Check sheet for the drawn part. Datum: minimum x, y, z corner. Units: mm. Coordinates: 2 decimals unless noted, no trailing zeros. Write each loop counter-clockwise with the first axis right and the second up, starting at its lowest first coordinate (ties: lowest second). Pieces come first, ordered by that corner, then holes. Notation, with made-up numbers: (-33, 88.25) -> (-19, 88.25) arc R29 cw to (-19, 116.25) -> close; hole circle Ø1 at (28.25, -24.75). An arc over 180 degrees is marked (long way). Answer in a Markdown table with one row per item. Add a question column.
Q1. Release check for a two-part mould opening along X. For the marked faces 1 and 2 record: pulls with the +X half, pulls with the -X half, needs draft (parallel to the pull), parting line crosses it, or undercut.
Q2. Section check C-C, the plane x = 30. Record the boundary of the cut face in (y, z) (1 decimal).
Q3. Section check D-D, the plane z = 1.5. Record the boundary of the cut face in (x, y) (1 decimal).
Q4. Thickness scan on line 1 (X direction, y = 12, z = 2.2) (1 decimal); line 2 (Y direction, x = 43, z = 0.35); line 3 (Y direction, x = 30, z = 2.8) (1 decimal). Record the ranges inside material, lowest first.
Q5. Gauge pin test, flat end, axial feed: P1, Ø8.5, axis at x = 29, y = 10, coming from the +Z side. Record the tip position at first contact, or that the pin passes through.
Q6. Section check A-A, the plane x = 43. Record the boundary of the cut face in (y, z).
Q7. Section check B-B, the plane y = 12. Record the boundary of the cut face in (x, z) (1 decimal).
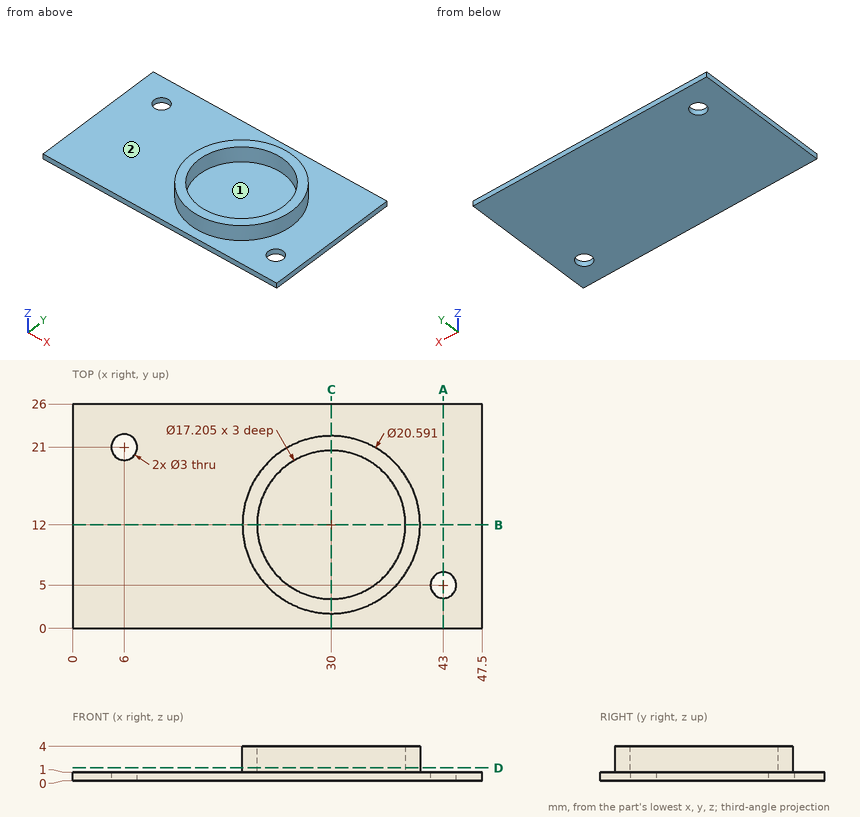
Calculated:
| question | item | result |
|---|---|---|
| 1 | face 1 | undercut |
| 1 | face 2 | needs draft |
| 2 | outline | (0, 0) -> (26, 0) -> (26, 1) -> (22.3, 1) -> (22.3, 4) -> (20.6, 4) -> (20.6, 1) -> (3.4, 1) -> (3.4, 4) -> (1.7, 4) -> (1.7, 1) -> (0, 1) -> close |
| 3 | outline | circle Ø20.6 at (30, 12); hole circle Ø17.2 at (30, 12) |
| 4 | line 1 | x = 19.7 to 21.4, 38.6 to 40.3 |
| 4 | line 2 | y = 0 to 3.5, 6.5 to 26 |
| 4 | line 3 | y = 1.7 to 3.4, 20.6 to 22.3 |
| 5 | P1 | stops at z = 1 |
| 6 | outline | (0, 0) -> (3.5, 0) -> (3.5, 1) -> (0, 1) -> close; (6.5, 0) -> (26, 0) -> (26, 1) -> (6.5, 1) -> close |
| 7 | outline | (0, 0) -> (47.5, 0) -> (47.5, 1) -> (40.3, 1) -> (40.3, 4) -> (38.6, 4) -> (38.6, 1) -> (21.4, 1) -> (21.4, 4) -> (19.7, 4) -> (19.7, 1) -> (0, 1) -> close |
